Work out the finished part from the listing and answer in its coordinate system (mm). Face numbers are marked on the shaded views. Give positions to 0.01 mm unless a question says otherwise; leave off trailing zeros. Loops run counter-clockwise (first coordinate to the right, second up) from the corner with the lowest first, then second, coordinate; pieces in that order, holes last. Notation, with made-up numbers: (-22.75, 57.25) -> (25.25, 57.25) arc R23 ccw to (25.25, 75.25) -> close; hole circle Ø2 at (-26, -29). An arc over 180 degrees is marked (long way). Answer as CSV lines item,"result". Start each with the question number.
1. Find section A-A, the plane x = 18. Give the vertices of the cut face in (y, z).
2. Determine the mould class of the marked faces 1 and 2 for opening direction X: +X half, -X half, draft (parallel to the pull), parting line (faces both ways), or undercut.
3. Find section D-D, the plane z = 32. Give the vertices of the cut face in (x, y).
4. Flat-ended cylindrical pins translate along their axes: pin 1 Ø2 at (y, z) = (-22.5, 1) entering from -X; pin 2 Ø12 at (x, y) = (-4.5, -54.5) entering from +Z; pin 3 Ø2.5 at (x, y) = (25.5, -40) entering from +Z. Find the tip coordinate at first contact, or state that the pin passes through.
5. Find section C-C, the plane y = 0. Give the vertices of the cut face in (x, z), and give its area (3 significant figures).
6. Find the intervals of material crossed by line 1 along Y through (x, z) = (-16.5, 11); line 2 along Y through (x, z) = (39.5, 11), in increasing order.
7. Find section B-B, the plane z = 7.5. Give the vertices of the cut face in (x, y).
from build123d import *

# Parameters (mm, degrees)
F5_R      = 2.5
F6_DEPTH  = 2
F7_DEPTH  = 34.5
F8_DEPTH  = 37.5
F9_DEPTH  = 17
F10_DEPTH = 20
F12_W     = 7.5
F12_H     = 32
F12_H_2   = 25
F13_DEPTH = 2


with BuildPart() as f6:
    # F5 (on Top) → F6 (new body)
    with BuildSketch(Plane.XY):
        with BuildLine():
            ThreePointArc((0, 4), (2.8284271247, 2.8284271247), (4, 0))
            ThreePointArc((4, 0), (2.8284271247, -2.8284271247), (0, -4))
            Line((0, -4), (42.5, -4))
            ThreePointArc((42.5, -4), (38.5, 0), (42.5, 4))
            Line((42.5, 4), (0, 4))
        make_face()
        with BuildLine():
            ThreePointArc((0, -4), (2.8284271247, -2.8284271247), (4, 0))
            ThreePointArc((4, 0), (2.8284271247, 2.8284271247), (0, 4))
            ThreePointArc((0, 4), (-4, 0), (0, -4))
        make_face()
        Circle(F5_R, mode=Mode.SUBTRACT)
        with BuildLine():
            ThreePointArc((46.5, 0), (45.3284271247, 2.8284271247), (42.5, 4))
            ThreePointArc((42.5, 4), (38.5, 0), (42.5, -4))
            ThreePointArc((42.5, -4), (45.3284271247, -2.8284271247), (46.5, 0))
        make_face()
        with Locations((42.5, 0)):
            Circle(F5_R, mode=Mode.SUBTRACT)
        Circle(F5_R)
        with Locations((42.5, 0)):
            Circle(F5_R)
    extrude(amount=F6_DEPTH)

    # F5 (on Top) → F7 (join)
    with BuildSketch(Plane.XY):
        with BuildLine():
            ThreePointArc((0, -4), (2.8284271247, -2.8284271247), (4, 0))
            ThreePointArc((4, 0), (2.8284271247, 2.8284271247), (0, 4))
            ThreePointArc((0, 4), (-4, 0), (0, -4))
        make_face()
        Circle(F5_R, mode=Mode.SUBTRACT)
        with BuildLine():
            ThreePointArc((46.5, 0), (45.3284271247, 2.8284271247), (42.5, 4))
            ThreePointArc((42.5, 4), (38.5, 0), (42.5, -4))
            ThreePointArc((42.5, -4), (45.3284271247, -2.8284271247), (46.5, 0))
        make_face()
        with Locations((42.5, 0)):
            Circle(F5_R, mode=Mode.SUBTRACT)
        Circle(F5_R)
        with Locations((42.5, 0)):
            Circle(F5_R)
    extrude(amount=F7_DEPTH)

    # F5 (on Top) → F8 (join)
    with BuildSketch(Plane.XY):
        Circle(F5_R)
        with Locations((42.5, 0)):
            Circle(F5_R)
    extrude(amount=F8_DEPTH)



with BuildPart() as f6b:
    # F5 (on Top) → F6, piece 2 (new body)
    with BuildSketch(Plane.XY):
        with BuildLine():
            ThreePointArc((0, -36), (2.8284271247, -37.1715728753), (4, -40))
            ThreePointArc((4, -40), (2.8284271247, -42.8284271247), (0, -44))
            Line((0, -44), (42.5, -44))
            ThreePointArc((42.5, -44), (38.5, -40), (42.5, -36))
            Line((42.5, -36), (0, -36))
        make_face()
        with BuildLine():
            ThreePointArc((46.5, -40), (45.3284271247, -37.1715728753), (42.5, -36))
            ThreePointArc((42.5, -36), (38.5, -40), (42.5, -44))
            ThreePointArc((42.5, -44), (45.3284271247, -42.8284271247), (46.5, -40))
        make_face()
        with Locations((42.5, -40)):
            Circle(F5_R, mode=Mode.SUBTRACT)
        with BuildLine():
            ThreePointArc((0, -44), (2.8284271247, -42.8284271247), (4, -40))
            ThreePointArc((4, -40), (2.8284271247, -37.1715728753), (0, -36))
            ThreePointArc((0, -36), (-4, -40), (0, -44))
        make_face()
        with Locations((0, -40)):
            Circle(F5_R, mode=Mode.SUBTRACT)
        with Locations((0, -40)):
            Circle(F5_R)
        with Locations((42.5, -40)):
            Circle(F5_R)
    extrude(amount=F6_DEPTH)

    # F5 (on Top) → F9 (join)
    with BuildSketch(Plane.XY):
        with BuildLine():
            ThreePointArc((0, -44), (2.8284271247, -42.8284271247), (4, -40))
            ThreePointArc((4, -40), (2.8284271247, -37.1715728753), (0, -36))
            ThreePointArc((0, -36), (-4, -40), (0, -44))
        make_face()
        with Locations((0, -40)):
            Circle(F5_R, mode=Mode.SUBTRACT)
        with BuildLine():
            ThreePointArc((46.5, -40), (45.3284271247, -37.1715728753), (42.5, -36))
            ThreePointArc((42.5, -36), (38.5, -40), (42.5, -44))
            ThreePointArc((42.5, -44), (45.3284271247, -42.8284271247), (46.5, -40))
        make_face()
        with Locations((42.5, -40)):
            Circle(F5_R, mode=Mode.SUBTRACT)
        with Locations((0, -40)):
            Circle(F5_R)
        with Locations((42.5, -40)):
            Circle(F5_R)
    extrude(amount=F9_DEPTH)

    # F5 (on Top) → F10 (join)
    with BuildSketch(Plane.XY):
        with Locations((0, -40)):
            Circle(F5_R)
        with Locations((42.5, -40)):
            Circle(F5_R)
    extrude(amount=F10_DEPTH)


with BuildPart() as f6b_1:
    # F11: moved
    add(f6b.part.moved(Location((-16.25, 0, 0))))


with BuildPart() as f6_1:
    add(f6.part)

    add(f6b_1.part)  # F13 merges F6b
    # F12 (on Top) → F13 (join)
    with BuildSketch(Plane.XY):
        with Locations((8.1697826646, -20)):
            Rectangle(F12_W, F12_H)
        with Locations((-7.5, -56.5)):
            Rectangle(F12_W, F12_H_2)
    extrude(amount=F13_DEPTH)


solid = f6_1.part
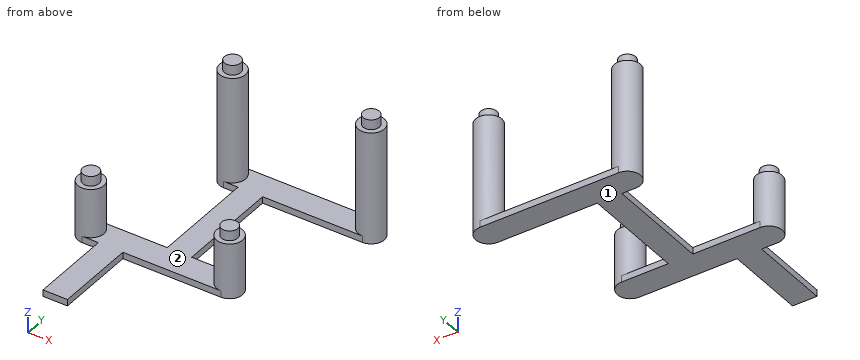
Resolved:
1,outline,"(-44, 0) -> (-36, 0) -> (-36, 2) -> (-44, 2) -> close; (-4, 0) -> (4, 0) -> (4, 2) -> (-4, 2) -> close"
2,face 1,"draft"
2,face 2,"undercut"
3,outline,"circle Ø8 at (0, 0); circle Ø8 at (42.5, 0)"
4,pin 1,"stops at x = 4.42"
4,pin 2,"stops at z = 2"
4,pin 3,"stops at z = 20"
5,outline,"(-4, 0) -> (46.5, 0) -> (46.5, 34.5) -> (45, 34.5) -> (45, 37.5) -> (40, 37.5) -> (40, 34.5) -> (38.5, 34.5) -> (38.5, 2) -> (4, 2) -> (4, 34.5) -> (2.5, 34.5) -> (2.5, 37.5) -> (-2.5, 37.5) -> (-2.5, 34.5) -> (-4, 34.5) -> close"
5,area,"651 mm^2"
6,line 1,"y = -43.99 to -36.01"
6,line 2,"y = -2.65 to 2.65"
7,outline,"circle Ø8 at (-16.25, -40); circle Ø8 at (0, 0); circle Ø8 at (26.25, -40); circle Ø8 at (42.5, 0)"
